CAD build for the part. Positions are in the model's coordinates, mm. A direction names the side the tool comes from. Coordinates: 2 decimals unless noted, no trailing zeros. Write each loop counter-clockwise with the first axis right and the second up, starting at its lowest first coordinate (ties: lowest second). Pieces come first, ordered by that corner, then holes.
```python
from build123d import *

# Parameters (mm, degrees)
BOSS_EXTRUDE1_DEPTH  = 12.7
FILLET1_R            = 6.35
M3_CLEARANCE_HOLE1_D = 3.4


with BuildPart() as part:
    # Sketch2 → Boss-Extrude1 (new body)
    with BuildSketch(Plane.XY):
        with BuildLine():
            Line((-34.671, -20.955), (-34.671, -35.371495007))
            ThreePointArc((-34.671, -35.371495007), (-18.725260376, -45.85395865), (0, -49.53))
            Line((0, -49.53), (0, -40.005))
            Line((0, -40.005), (-21.971, -40.005))
            Line((-21.971, -40.005), (-21.971, -30.909518363))
            Line((-21.971, -30.909518363), (-26.940768363, -30.909518363))
            ThreePointArc((-26.940768363, -30.909518363), (-30.909518363, -26.940768363), (-26.940768363, -22.972018363))
            Line((-26.940768363, -22.972018363), (-21.971, -22.972018363))
            Line((-21.971, -22.972018363), (-21.971, -20.955))
            Line((-21.971, -20.955), (-34.671, -20.955))
        make_face()
    boss_extrude1 = extrude(amount=BOSS_EXTRUDE1_DEPTH)

    # Mirror1: Boss-Extrude1 across plane
    add(boss_extrude1.mirror(Plane(origin=(0, -40.005, 12.7), x_dir=(0, 0, 1), z_dir=(-1, 0, 0))))

    # Fillet1
    fillet1_edges = [part.edges().sort_by_distance(p)[0] for p in [
        (-34.671, -20.955, 6.35),
        (34.671, -20.955, 6.35),
    ]]
    fillet(fillet1_edges, radius=FILLET1_R)

    # M3 Clearance Hole1 (through all)
    with Locations(Plane.XY.offset(12.7)):
        with Locations((0, -44.45)):
            Hole(M3_CLEARANCE_HOLE1_D / 2)


solid = part.part
```
Item 1: Wall check: line 1 along Y through (x, z) = (0, 7) (3 decimals); line 2 along X through (y, z) = (-31.5, 3.5); line 3 along X through (y, z) = (-27, 7). Give the ranges that are in metal, low to high.
Item 2: Saw through at D-D, the plane x = -12.5. Write the cut outline in (y, z) (3 decimals), and give its area (3 significant figures).
Item 3: Saw through at A-A, the plane y = -36.5. Write the cut outline in (x, z), and give its area (3 significant figures).
Item 4: Which spindle directions (+Z, -Z, +X, -X, +Y, -Y) get a long thin tool onto all of the face, cutting with end or side? Do faces 1 (the flat face through (0, -41, 12.7)), 2 (the flat face through (21.971, -36, 6)), 3 (the flat face through (24, -30.91, 6)). Say none if no direction does.
Item 5: Flat gauge pins, fed straight in: pin 1 Ø5.5 at (x, z) = (-24, 8) entering from -Y; pin 2 Ø0.6 at (y, z) = (-21.5, 5) entering from +X; pin 3 Ø5 at (x, z) = (24, 11.5) entering from -Y; pin 4 Ø5 at (y, z) = (-36, 8.5) entering from +X. Where does each tip first touch, or does it go through?
Item 6: Saw through at C-C, the plane y = -44.45. Write the cut outline in (x, z), and give its area (3 significant figures).
Item 7: Two-plate mould, pull along X, no slides. Class faces 4 (the flat face through (-34.671, -31, 6)), 5 (the flat face through (-21.971, -22, 6)), 6 (the flat face through (-25, -20.955, 6)): +X half, -X half, draft (parallel to the pull), parting line (faces both ways), or undercut.
Working result:
1. line 1: y = -49.53 to -46.15, -42.75 to -40.005
1. line 2: x = -34.67 to -21.97, 21.97 to 34.67
1. line 3: x = -34.66 to -30.91, 30.91 to 34.66
2. outline: (-47.927, 0) - (-40.005, 0) - (-40.005, 12.7) - (-47.927, 12.7) - close
2. area: 101 mm2
3. outline: (-33.48, 0) - (-21.97, 0) - (-21.97, 12.7) - (-33.48, 12.7) - close; (21.97, 0) - (33.48, 0) - (33.48, 12.7) - (21.97, 12.7) - close
3. area: 292 mm2
4. face 1: +Z, +X, -X, +Y, -Y
4. face 2: +Z, -Z, +Y
4. face 3: +Z, -Z
5. pin 1: stops at y = -44.74
5. pin 2: stops at x = 31.49
5. pin 3: stops at y = -44.62
5. pin 4: stops at x = 34.67
6. outline: (-21.85, 0) - (-1.7, 0) - (-1.7, 12.7) - (-21.85, 12.7) - close; (1.7, 0) - (21.85, 0) - (21.85, 12.7) - (1.7, 12.7) - close
6. area: 512 mm2
7. face 4: -X half
7. face 5: undercut
7. face 6: draft
